Geometry check sheet. Reference: the model listing, model coordinates, mm. Face numbers are marked on the shaded views. A direction names the side the tool comes from. Coordinates: 2 decimals unless noted, no trailing zeros. Order: outer loops, then holes, each group sorted by start corner. A loop starts at its lowest first (then second) coordinate and runs counter-clockwise, first axis right, second up. Notation, with made-up numbers: (-38, 59.5) -> (-1, 59.5) arc R29 ccw to (-1, 89.5) -> close; hole circle Ø10 at (84, 64). An arc over 180 degrees is marked (long way). Answer as CSV lines item,"result". Start each with the question number.
from build123d import *

# Parameters (mm, degrees)
SKETCH2_R           = 27.5
BOSS_EXTRUDE1_DEPTH = 65.024
SKETCH3_W           = 85
SKETCH3_H           = 230
BOSS_EXTRUDE2_DEPTH = 13.716
SKETCH4_W           = 43.394113748
SKETCH4_H           = 7
SKETCH4_W_2         = 45.361068276
BOSS_EXTRUDE3_DEPTH = 41
SKETCH7_R           = 18.75
CUT_EXTRUDE3_DEPTH  = 65.024
SKETCH5_R           = 21
CUT_EXTRUDE1_DEPTH  = 21
SKETCH6_R           = 23.5
CUT_EXTRUDE2_DEPTH  = 15
CUT_EXTRUDE4_START  = -25
SKETCH8_R           = 21
CUT_EXTRUDE4_DEPTH  = 25
SKETCH10_W          = 8
SKETCH10_H          = 170
BOSS_EXTRUDE4_DEPTH = 35
CUT_EXTRUDE5_REACH  = 159.093
CUT_EXTRUDE6_REACH  = 209.583
SKETCH14_R          = 3.898215838
BOSS_EXTRUDE5_START = 15
BOSS_EXTRUDE5_DEPTH = 10
SKETCH21_W          = 19
SKETCH21_H          = 6
BOSS_EXTRUDE6_DEPTH = 38
CUT_EXTRUDE7_REACH  = 178.644
SKETCH22_R          = 4


with BuildPart() as part:
    # Sketch2 → Boss-Extrude1 (new body)
    with BuildSketch(Plane.XY):
        Circle(SKETCH2_R)
    extrude(amount=BOSS_EXTRUDE1_DEPTH)

    # Sketch3 → Boss-Extrude2 (add)
    with BuildSketch(Plane.XY):
        Rectangle(SKETCH3_W, SKETCH3_H)
    extrude(amount=BOSS_EXTRUDE2_DEPTH)

    # Sketch4 → Boss-Extrude3 (add)
    with BuildSketch(Plane.XY.offset(13.716)):
        with Locations((0, -106)):
            Rectangle(SKETCH4_W, SKETCH4_H)
        with Locations((0, -81)):
            Rectangle(SKETCH4_W_2, SKETCH4_H)
    extrude(amount=BOSS_EXTRUDE3_DEPTH)

    # Sketch7 → Cut-Extrude3 (cut)
    with BuildSketch(Plane.XY.offset(65.024)):
        Circle(SKETCH7_R)
    extrude(amount=-CUT_EXTRUDE3_DEPTH, mode=Mode.SUBTRACT)

    # Sketch5 → Cut-Extrude1 (cut)
    with BuildSketch(Plane.XY.offset(65.024)):
        Circle(SKETCH5_R)
    extrude(amount=-CUT_EXTRUDE1_DEPTH, mode=Mode.SUBTRACT)

    # Sketch6 → Cut-Extrude2 (cut)
    with BuildSketch(Plane(origin=(0, 0, 0), x_dir=(-1, 0, 0), z_dir=(0, 0, -1))):
        Circle(SKETCH6_R)
    extrude(amount=-CUT_EXTRUDE2_DEPTH, mode=Mode.SUBTRACT)

    # Sketch8 → Cut-Extrude4 (cut)
    with BuildSketch(Plane(origin=(0, 0, 0), x_dir=(-1, 0, 0), z_dir=(0, 0, -1)).offset(CUT_EXTRUDE4_START)):
        with Locations(Location((0, 0, 0), (0, 0, 180))):
            Circle(SKETCH8_R)
    extrude(amount=CUT_EXTRUDE4_DEPTH, mode=Mode.SUBTRACT)

    # Sketch10 → Boss-Extrude4 (add)
    with BuildSketch(Plane.XY.offset(13.716)):
        with Locations((-38.5, 0)):
            Rectangle(SKETCH10_W, SKETCH10_H)
        with Locations((38.5, 0)):
            Rectangle(SKETCH10_W, SKETCH10_H)
    extrude(amount=BOSS_EXTRUDE4_DEPTH)

    # Cut-Extrude5: up to this face of the body (flat: up to its plane)
    cut_extrude5_end = Plane(part.part.faces().sort_by_distance((42.5, 0, 22.776198113))[0])
    # Sketch11 → Cut-Extrude5 (cut, up to the picked face)
    with BuildSketch(Plane.ZY.offset(42.5), mode=Mode.PRIVATE) as cut_extrude5_sk1:
        Polygon((13.716, 85), (48.716, 50), (48.716, 85), align=None)
    cut_extrude5_tool1 = split(extrude(cut_extrude5_sk1.sketch, amount=-CUT_EXTRUDE5_REACH, mode=Mode.PRIVATE), bisect_by=cut_extrude5_end, keep=Keep.BOTH, mode=Mode.PRIVATE)
    add(cut_extrude5_tool1.solids().sort_by(Axis((-42.5, 73.333333, 37.049333), (1, 0, 0)))[0], mode=Mode.SUBTRACT)

    # Cut-Extrude6: up to this face of the body (flat: up to its plane)
    cut_extrude6_end = Plane(part.part.faces().sort_by_distance((0, -109.5, 34.216))[0])
    # Sketch14 → Cut-Extrude6 (cut, up to the picked face)
    with BuildSketch(Plane(origin=(0, -77.5, 0), x_dir=(1, 0, 0), z_dir=(0, 1, 0)), mode=Mode.PRIVATE) as cut_extrude6_sk1:
        with Locations(Location((-6.143911141, -38.35, 0), (0, 0, 270))):
            Circle(SKETCH14_R)
    cut_extrude6_tool1 = split(extrude(cut_extrude6_sk1.sketch, amount=-CUT_EXTRUDE6_REACH, mode=Mode.PRIVATE), bisect_by=cut_extrude6_end, keep=Keep.BOTH, mode=Mode.PRIVATE)
    add(cut_extrude6_tool1.solids().sort_by(Axis((-6.143911, -77.5, 38.35), (0, -1, 0)))[0], mode=Mode.SUBTRACT)

    # Sketch16 → Boss-Extrude5 (add)
    with BuildSketch(Plane.XY.offset(BOSS_EXTRUDE5_START)):
        Polygon((78.5, -42), (42.5, -15), (42.5, -69), align=None)
        Polygon((42.5, 69), (78.5, 42), (42.5, 15), align=None)
    extrude(amount=BOSS_EXTRUDE5_DEPTH)

    # Sketch21 → Boss-Extrude6 (add)
    with BuildSketch(Plane.ZY.offset(42.5)):
        with Locations((25.65, -53.16)):
            Rectangle(SKETCH21_W, SKETCH21_H)
        with Locations((25.65, -31.16)):
            Rectangle(SKETCH21_W, SKETCH21_H)
    extrude(amount=BOSS_EXTRUDE6_DEPTH)

    # Cut-Extrude7: up to this face of the body (flat: up to its plane)
    cut_extrude7_end = Plane(part.part.faces().sort_by_distance((-61.5, -56.16, 25.65))[0])
    # Sketch22 → Cut-Extrude7 (cut, up to the picked face)
    with BuildSketch(Plane(origin=(0, -28.16, 0), x_dir=(1, 0, 0), z_dir=(0, 1, 0)), mode=Mode.PRIVATE) as cut_extrude7_sk1:
        with Locations(Location((-69.643911141, -25.65, 0), (0, 0, 180))):
            Circle(SKETCH22_R)
    cut_extrude7_tool1 = split(extrude(cut_extrude7_sk1.sketch, amount=-CUT_EXTRUDE7_REACH, mode=Mode.PRIVATE), bisect_by=cut_extrude7_end, keep=Keep.BOTH, mode=Mode.PRIVATE)
    add(cut_extrude7_tool1.solids().sort_by(Axis((-69.643911, -28.16, 25.65), (0, -1, 0)))[0], mode=Mode.SUBTRACT)


solid = part.part
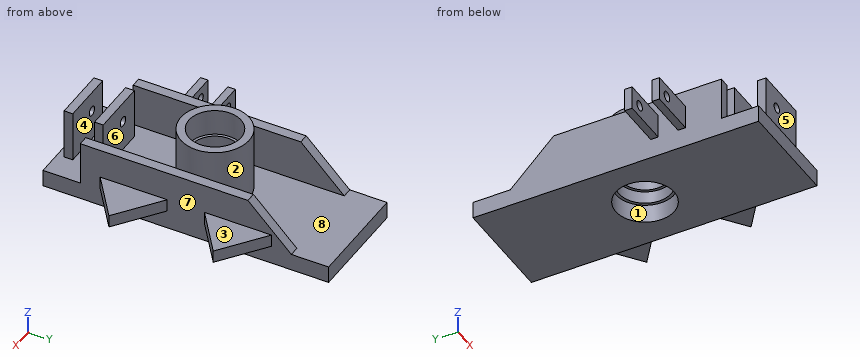
Q1. Thickness scan on L1, parallel to X at y = -51.5, z = 26; L2, parallel to Y at x = 0, z = 57; L3, parallel to X at y = 43, z = 38.5. Record the ranges inside material, lowest first.
Q2. Go/stop test with flat-tipped pins: pin 1 Ø8 at (x, z) = (18.5, 26.5) entering from -Y; pin 2 Ø6 at (x, z) = (28, 39) entering from -Y; pin 3 Ø18 at (x, y) = (58.5, -48) entering from -Z; pin 4 Ø1.5 at (x, y) = (-42.5, -67) entering from -Z. Record where each tip stops, or that it passes through.
Q3. Sectioned sample at A-A, the plane y = 0. Record the cut outline in (x, z), then the cut area to 3 significant figures.
Q4. Access from +Z, -Z, +X, -X, +Y, -Y to the whole of each face (thin tool, end or side, straight path). Record for the marked faces 1, 2, 3 and 4.
Q5. Sectioned sample at D-D, the plane y = 45. Record the cut outline in (x, z).
Q6. Sectioned sample at B-B, the plane z = 38.35. Record the cut outline in (x, y).
Q7. Release check for a two-part mould opening along X. For the marked faces 5, 6, 7 and 8 record: released by +X, released by -X, zero draft, split by the parting line, or undercut.
Geometry results:
1,L1,"x = -80.5 to -73.63, -65.66 to -34.5, 34.5 to 42.5"
1,L2,"y = -27.5 to -21, 21 to 27.5"
1,L3,"x = -42.5 to -34.5, 34.5 to 42.5"
2,pin 1,"stops at y = -109.5"
2,pin 2,"stops at y = -11.46"
2,pin 3,"stops at z = 15"
2,pin 4,"stops at z = 0"
3,outline,"(-42.5, 0) -> (-23.5, 0) -> (-23.5, 15) -> (-21, 15) -> (-21, 25) -> (-18.75, 25) -> (-18.75, 44.02) -> (-21, 44.02) -> (-21, 65.02) -> (-27.5, 65.02) -> (-27.5, 13.72) -> (-34.5, 13.72) -> (-34.5, 48.72) -> (-42.5, 48.72) -> close; (18.75, 25) -> (21, 25) -> (21, 15) -> (23.5, 15) -> (23.5, 0) -> (42.5, 0) -> (42.5, 48.72) -> (34.5, 48.72) -> (34.5, 13.72) -> (27.5, 13.72) -> (27.5, 65.02) -> (21, 65.02) -> (21, 44.02) -> (18.75, 44.02) -> close"
3,area,"1,830 mm^2"
4,face 1,"-Z"
4,face 2,"+Z"
4,face 3,"+Z, +X, +Y, -Y"
4,face 4,"+Z, +X, -X"
5,outline,"(-42.5, 0) -> (42.5, 0) -> (42.5, 15) -> (74.5, 15) -> (74.5, 25) -> (42.5, 25) -> (42.5, 48.72) -> (34.5, 48.72) -> (34.5, 13.72) -> (-34.5, 13.72) -> (-34.5, 48.72) -> (-42.5, 48.72) -> close"
6,outline,"(-42.5, -85) -> (-34.5, -85) -> (-34.5, 60.37) -> (-42.5, 60.37) -> close; circle Ø55 at (0, 0); (-22.68, -84.5) -> (-10.04, -84.5) -> (-10.04, -77.5) -> (-22.68, -77.5) -> close; (-21.7, -109.5) -> (-10.04, -109.5) -> (-10.04, -102.5) -> (-21.7, -102.5) -> close; (-2.25, -109.5) -> (21.7, -109.5) -> (21.7, -102.5) -> (-2.25, -102.5) -> close; (-2.25, -84.5) -> (22.68, -84.5) -> (22.68, -77.5) -> (-2.25, -77.5) -> close; (34.5, -85) -> (42.5, -85) -> (42.5, 60.37) -> (34.5, 60.37) -> close; hole circle Ø37.5 at (0, 0)"
7,face 5,"zero draft"
7,face 6,"undercut"
7,face 7,"released by +X"
7,face 8,"undercut"
